Build history of the part. All positions in model axes, mm. Face numbers are marked on the shaded views. A direction names the side the tool comes from. Give positions to 0.01 mm unless a question says otherwise; leave off trailing zeros. Write each loop counter-clockwise with the first axis right and the second up, starting at its lowest first coordinate (ties: lowest second). Pieces come first, ordered by that corner, then holes. Notation, with made-up numbers: M 43.5,68 L 98.5,68 A11 cw 98.5,88 Z; hole C 78.5,20 d3. An arc over 180 degrees is marked long. One line per item, written item: value. Start each with the question number.
from build123d import *

# Parameters (mm, degrees)
ESBO_O1_W                  = 2.8
ESBO_O1_H                  = 2.8
RESSALTO_EXTRUS_O1_DEPTH   = 16
CORTE_EXTRUS_O_FINA1_START = -11
CORTE_EXTRUS_O_FINA1_DEPTH = 11


with BuildPart() as part:
    # Esboço1 → Ressalto-extrusão1 (new body)
    with BuildSketch(Plane.XY):
        with BuildLine():
            ThreePointArc((2.870828693, 8.870828693), (-1.470083208, 10.615120525), (-2.236067977, 6))
            ThreePointArc((-2.236067977, 6), (-1.472135955, 4), (-2.236067977, 2))
            ThreePointArc((-2.236067977, 2), (-2.121320344, -2.121320344), (2, -2.236067977))
            ThreePointArc((2, -2.236067977), (4, -1.472135955), (6, -2.236067977))
            ThreePointArc((6, -2.236067977), (10.615120525, -1.470083208), (8.870828693, 2.870828693))
            ThreePointArc((8.870828693, 2.870828693), (7.620337043, 3.620337043), (6.870828693, 4.870828693))
            ThreePointArc((6.870828693, 4.870828693), (6.121320344, 6.121320344), (4.870828693, 6.870828693))
            ThreePointArc((4.870828693, 6.870828693), (3.620337043, 7.620337043), (2.870828693, 8.870828693))
        make_face()
        with Locations((0, 8)):
            Rectangle(ESBO_O1_W, ESBO_O1_H, mode=Mode.SUBTRACT)
        Polygon((4, 5.979898987), (5.979898987, 4), (4, 2.020101013), (2.020101013, 4), align=None, mode=Mode.SUBTRACT)
        with Locations((8, 0)):
            Rectangle(ESBO_O1_W, ESBO_O1_H, mode=Mode.SUBTRACT)
        Rectangle(ESBO_O1_W, ESBO_O1_H, mode=Mode.SUBTRACT)
    extrude(amount=RESSALTO_EXTRUS_O1_DEPTH)

    # Esboço2 → Corte-Extrusão-Fina1 (cut)
    with BuildSketch(Plane.XY.offset(16).offset(CORTE_EXTRUS_O_FINA1_START)):
        with BuildLine():
            Line((9.333446825, -9.049130918), (14.39222363, -3.094607445))
            ThreePointArc((14.39222363, -3.094607445), (13.208027354, 13.176721236), (-3.059004987, 14.418541135))
            Line((-3.059004987, 14.418541135), (-8.835216439, 9.536191613))
            ThreePointArc((-8.835216439, 9.536191613), (-9.295999773, -9.087595294), (9.333446825, -9.049130918))
        make_face()
        with BuildLine():
            Line((2, -2.236067977), (6.47600505, 3.032493606))
            ThreePointArc((6.47600505, 3.032493606), (6.125574464, 6.117055961), (3.04273657, 6.482346303))
            Line((3.04273657, 6.482346303), (-2.144816713, 2.09756079))
            ThreePointArc((-2.144816713, 2.09756079), (-2.16802388, -2.073565156), (2, -2.236067977))
        make_face(mode=Mode.SUBTRACT)
    extrude(amount=CORTE_EXTRUS_O_FINA1_DEPTH, mode=Mode.SUBTRACT)


solid = part.part
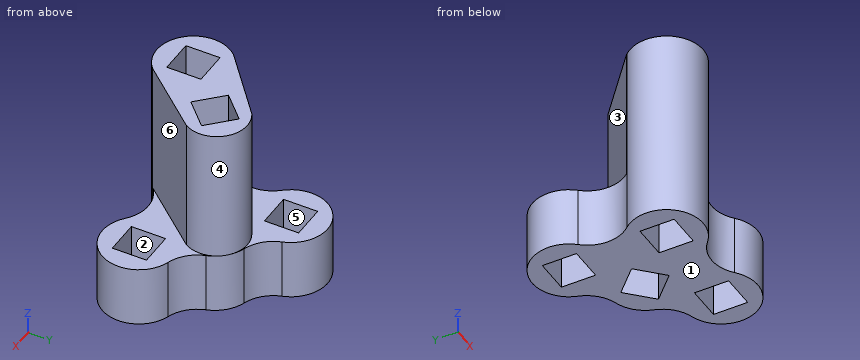
1) Band-saw the part on B-B (z = 5.25). List the corners of the cut face in (x, y), then the cut area to 3 significant figures.
2) Band-saw the part on A-A (z = 2.75). List the corners of the cut face in (x, y).
3) Drop flat-ended pins along their axis: P1, Ø2, axis at x = 7.5, y = 7, coming from the +Z side; P2, Ø1, axis at x = 2.5, z = 9.5, coming from the +Y side; P3, Ø0.8, axis at y = -0.5, z = 5.5, coming from the +X side; P4, Ø1.4, axis at x = 8, z = 2, coming from the +Y side. Give the stop position or say it passes through.
4) Band-saw the part on C-C (x = 4.5). List the corners of the cut face in (y, z), then the cut area to 3 significant figures.
5) Band-saw the part on D-D (y = 0). List the corners of the cut face in (x, z), then the cut area to 3 significant figures.
6) Tool access for the marked faces 1, 2 and 3: list every direction of +Z, -Z, +X, -X, +Y, -Y with a clear straight run to the whole face (end or side of a thin tool).
7) Probe line 1 along X through (y, z) = (0.25, 2.75); line 2 along Z through (x, y) = (-1.25, 3); line 3 along X through (y, z) = (9, 2). List the from-to ranges inside material, lowest first. Write a range as from..to.
8) Mould opens along X. For the marked faces 4, 5 and 6 say: released by +X, released by -X, zero draft, split by the parting line, or undercut.
Model answer:
1. outline: M -2.14,2.1 A3 ccw 2,-2.24 L 6.48,3.03 A2.5 ccw 3.04,6.48 Z; hole M -1.4,-1.4 L 1.4,-1.4 L 1.4,1.4 L -1.4,1.4 Z; hole M 2.02,4 L 4,2.02 L 5.98,4 L 4,5.98 Z
1. area: 41.9 mm²
2. outline: M -2.24,2 A3 ccw 2,-2.24 A3 cw 6,-2.24 A3 ccw long 8.87,2.87 A3 cw 6.87,4.87 A3 ccw 4.87,6.87 A3 cw 2.87,8.87 A3 ccw long -2.24,6 A3 cw Z; hole M -1.4,-1.4 L 1.4,-1.4 L 1.4,1.4 L -1.4,1.4 Z; hole M -1.4,6.6 L 1.4,6.6 L 1.4,9.4 L -1.4,9.4 Z; hole M 2.02,4 L 4,2.02 L 5.98,4 L 4,5.98 Z; hole M 6.6,-1.4 L 9.4,-1.4 L 9.4,1.4 L 6.6,1.4 Z
3. P1: passes through
3. P2: stops at y = 6.45
3. P3: stops at x = 3.81
3. P4: stops at y = 4
4. outline: M -1.51,0 L 2.52,0 L 2.52,16 L 0.71,16 L 0.71,5 L -1.51,5 Z; M 5.48,0 L 7.01,0 L 7.01,5 L 6.85,5 L 6.85,16 L 5.48,16 Z
4. area: 62.8 mm²
5. outline: M -3,0 L -1.4,0 L -1.4,16 L -3,16 Z; M 1.4,0 L 6.6,0 L 6.6,5 L 3.9,5 L 3.9,16 L 1.4,16 Z; M 9.4,0 L 11,0 L 11,5 L 9.4,5 Z
5. area: 87.1 mm²
6. face 1: -Z, +X, -X, +Y, -Y
6. face 2: +Z, -Z
6. face 3: +Z, -X, +Y
7. line 1: x = -2.99..-1.4, 1.4..6.6, 9.4..10.99
7. line 2: z = 0..5
7. line 3: x = -2.83..-1.4, 1.4..2.83
8. face 4: split by the parting line
8. face 5: undercut
8. face 6: released by +X
